Source: CAD feature listing. Evaluate the final solid. Frame: model axes, mm. A direction names the side the tool comes from. Give positions to 0.01 mm unless a question says otherwise; leave off trailing zeros. Loops run counter-clockwise (first coordinate to the right, second up) from the corner with the lowest first, then second, coordinate; pieces in that order, holes last. Notation, with made-up numbers: (4, 51) -> (22, 51) arc R10 cw to (22, 60) -> close; hole circle Ø7 at (55.25, 35). An arc over 180 degrees is marked (long way). Put each result on its own line as item: value.
```python
from build123d import *

# Parameters (mm, degrees)
SKETCH2_R             = 1.6
BOSS_EXTRUDE1_DEPTH   = 2
BOSS_EXTRUDE1_2_DEPTH = 2
BOSS_EXTRUDE2_DEPTH   = 12.7
SKETCH4_R             = 1.8
BOSS_EXTRUDE3_DEPTH   = 2
CHAMFER1_SIZE         = 2.54


with BuildPart() as part:
    # Sketch2 → Boss-Extrude1 (new body)
    with BuildSketch(Plane(origin=(0, 84.355025863, 0), x_dir=(1, 0, 0), z_dir=(0, 1, 0))):
        with BuildLine():
            Line((86.165130669, -169.940155685), (88.815130669, -169.940155685))
            ThreePointArc((88.815130669, -169.940155685), (90.611181893, -169.196206909), (91.355130669, -167.400155685))
            Line((91.355130669, -167.400155685), (91.355130669, -166.020155685))
            Line((91.355130669, -166.020155685), (94.293130669, -166.020155685))
            Line((94.293130669, -166.020155685), (94.293130669, -163.082155685))
            Line((94.293130669, -163.082155685), (94.293130669, -156.732155685))
            Line((94.293130669, -156.732155685), (86.165130669, -156.732155685))
            ThreePointArc((86.165130669, -156.732155685), (84.369079444, -157.47610446), (83.625130669, -159.272155685))
            Line((83.625130669, -159.272155685), (83.625130669, -167.400155685))
            ThreePointArc((83.625130669, -167.400155685), (84.369079444, -169.196206909), (86.165130669, -169.940155685))
        make_face()
        with Locations(Location((86.773356517, -166.898975693, 0), (0, 0, 270))):
            Circle(SKETCH2_R, mode=Mode.SUBTRACT)
        with Locations(Location((89.895511725, -160.090079663, 0), (0, 0, 270))):
            Circle(SKETCH2_R, mode=Mode.SUBTRACT)
    extrude(amount=BOSS_EXTRUDE1_DEPTH)



with BuildPart() as body_2:
    # Sketch2 → Boss-Extrude1 2 (new body)
    with BuildSketch(Plane(origin=(0, 84.355025863, 0), x_dir=(1, 0, 0), z_dir=(0, 1, 0))):
        with BuildLine():
            Line((113.995130669, -169.940155685), (116.645130669, -169.940155685))
            ThreePointArc((116.645130669, -169.940155685), (118.441181893, -169.196206909), (119.185130669, -167.400155685))
            Line((119.185130669, -167.400155685), (119.185130669, -159.272155685))
            ThreePointArc((119.185130669, -159.272155685), (118.441181893, -157.47610446), (116.645130669, -156.732155685))
            Line((116.645130669, -156.732155685), (108.517130669, -156.732155685))
            Line((108.517130669, -156.732155685), (108.517130669, -163.082155685))
            Line((108.517130669, -163.082155685), (108.517130669, -166.020155685))
            Line((108.517130669, -166.020155685), (111.455130669, -166.020155685))
            Line((111.455130669, -166.020155685), (111.455130669, -167.400155685))
            ThreePointArc((111.455130669, -167.400155685), (112.199079444, -169.196206909), (113.995130669, -169.940155685))
        make_face()
        with Locations(Location((116.03690482, -166.898975693, 0), (0, 0, 270))):
            Circle(SKETCH2_R, mode=Mode.SUBTRACT)
        with Locations(Location((112.914749612, -160.090079663, 0), (0, 0, 270))):
            Circle(SKETCH2_R, mode=Mode.SUBTRACT)
    extrude(amount=BOSS_EXTRUDE1_2_DEPTH)


with BuildPart() as part_1:
    add(part.part)

    add(body_2.part)  # Boss-Extrude2 merges body 2
    # Sketch3 → Boss-Extrude2 (add)
    with BuildSketch(Plane(origin=(0, 86.355025863, 0), x_dir=(1, 0, 0), z_dir=(0, 1, 0))):
        with BuildLine():
            Line((108.517130669, -158.002155685), (108.517130669, -156.732155685))
            Line((108.517130669, -156.732155685), (94.293130669, -156.732155685))
            Line((94.293130669, -156.732155685), (86.165130669, -156.732155685))
            ThreePointArc((86.165130669, -156.732155685), (84.369079444, -157.47610446), (83.625130669, -159.272155685))
            Line((83.625130669, -159.272155685), (83.625130669, -164.352155685))
            Line((83.625130669, -164.352155685), (87.435130669, -164.352155685))
            Line((87.435130669, -164.352155685), (87.435130669, -158.002155685))
            Line((87.435130669, -158.002155685), (108.517130669, -158.002155685))
        make_face()
        with BuildLine():
            Line((115.375130669, -164.352155685), (119.185130669, -164.352155685))
            Line((119.185130669, -164.352155685), (119.185130669, -159.272155685))
            ThreePointArc((119.185130669, -159.272155685), (118.441181893, -157.47610446), (116.645130669, -156.732155685))
            Line((116.645130669, -156.732155685), (108.517130669, -156.732155685))
            Line((108.517130669, -156.732155685), (108.517130669, -158.002155685))
            Line((108.517130669, -158.002155685), (115.375130669, -158.002155685))
            Line((115.375130669, -158.002155685), (115.375130669, -164.352155685))
        make_face()
    extrude(amount=BOSS_EXTRUDE2_DEPTH)

    # Sketch4 → Boss-Extrude3 (add)
    with BuildSketch(Plane(origin=(0, 99.055025863, 0), x_dir=(1, 0, 0), z_dir=(0, 1, 0))):
        with BuildLine():
            Line((83.625130669, -164.352155685), (83.625130669, -191.022155685))
            Line((83.625130669, -191.022155685), (119.185130669, -191.022155685))
            Line((119.185130669, -191.022155685), (119.185130669, -164.352155685))
            Line((119.185130669, -164.352155685), (119.185130669, -159.272155685))
            ThreePointArc((119.185130669, -159.272155685), (118.441181893, -157.47610446), (116.645130669, -156.732155685))
            Line((116.645130669, -156.732155685), (86.165130669, -156.732155685))
            ThreePointArc((86.165130669, -156.732155685), (84.369079444, -157.47610446), (83.625130669, -159.272155685))
            Line((83.625130669, -159.272155685), (83.625130669, -164.352155685))
        make_face()
        with Locations(Location((93.405130669, -184.164155685, 0), (0, 0, 270))):
            Circle(SKETCH4_R, mode=Mode.SUBTRACT)
        with Locations(Location((109.405130669, -184.164155685, 0), (0, 0, 270))):
            Circle(SKETCH4_R, mode=Mode.SUBTRACT)
    extrude(amount=BOSS_EXTRUDE3_DEPTH)

    # Chamfer1
    chamfer1_edges = [part_1.edges().sort_by_distance(p)[0] for p in [
        (85.530130669, 99.055025863, 164.352155685),
        (87.435130669, 99.055025863, 161.177155685),
        (101.405130669, 99.055025863, 158.002155685),
        (115.375130669, 99.055025863, 161.177155685),
        (117.280130669, 99.055025863, 164.352155685),
    ]]
    chamfer(chamfer1_edges, length=CHAMFER1_SIZE)


solid = part_1.part
```
(1) Reachability of faces 1 (the cylindrical face through (114.6, 85.3, 167.6)), 2 (the flat face through (116.671, 97.803, 165.64)), 3 (the flat face through (88.72, 97.8, 162.51)), 4 (the cylindrical face through (90.591, 85.341, 169.216)), 5 (the flat face through (108.517, 85, 161)) from +Z, -Z, +X, -X, +Y, -Y: full face, straight path, thin tool, end or side. Return the list, or none.
Calculated:
face 1: -Y
face 2: +Z, +X, -X
face 3: +Z
face 4: +Z, -Y
face 5: +Z, -Z, -Y
(2) Line query: probe 1 along X at (y, z) = (99.25, 183); probe 2 along X at (y, z) = (89, 162.5); probe 3 along X at (y, z) = (85.5, 161.5). Output: solid intervals per line, ascending. Write a range as from..to.
Calculated:
probe 1: x = 83.63..92.03, 94.78..108.03, 110.78..119.19
probe 2: x = 83.63..87.44, 115.38..119.19
probe 3: x = 83.63..89.14, 90.65..94.29, 108.52..112.16, 113.67..119.19
(3) First-contact query: P1, Ø0.6, axis at x = 115.5, y = 85, coming from the +Z side; P2, Ø4, axis at x = 117, y = 91, coming from the +Z side; P3, Ø1, axis at x = 92, y = 90.5, coming from the +Z side; P4, Ø4, axis at x = 116.04, z = 166.9, coming from the -Y side (3 decimals). Flat tips, straight axial feed; report the tip coordinate or a pass-through.
Calculated:
P1: stops at z = 169.94
P2: stops at z = 164.35
P3: stops at z = 158
P4: stops at y = 84.355
(4) Section C-C on z = 169. Return loops of the section in (x, y).
Calculated:
outline: (83.63, 99.06) -> (119.19, 99.06) -> (119.19, 101.06) -> (83.63, 101.06) -> close; (84.19, 84.36) -> (90.79, 84.36) -> (90.79, 86.36) -> (84.19, 86.36) -> close; (112.02, 84.36) -> (118.62, 84.36) -> (118.62, 86.36) -> (112.02, 86.36) -> close
(5) Section A-A on y = 94.75. Return loops of the section in (x, z).
Calculated:
outline: (83.63, 159.27) arc R2.54 ccw to (86.17, 156.73) -> (116.65, 156.73) arc R2.54 ccw to (119.19, 159.27) -> (119.19, 164.35) -> (115.38, 164.35) -> (115.38, 158) -> (87.44, 158) -> (87.44, 164.35) -> (83.63, 164.35) -> close
(6) Section B-B on x = 103. Return loops of the section in (y, z).
Calculated:
outline: (86.36, 156.73) -> (101.06, 156.73) -> (101.06, 191.02) -> (99.06, 191.02) -> (99.06, 160.54) -> (96.52, 158) -> (86.36, 158) -> close
(7) Draft query along Z for faces 6 (the flat face through (101, 100, 191.022)), 7 (the flat face through (90, 86.355, 164)), 8 (the cylindrical face through (113.996, 85.341, 158.911)). Return one class per face: released by +Z, released by -Z, zero draft, split by the parting line, or undercut.
Calculated:
face 6: released by +Z
face 7: zero draft
face 8: undercut
(8) Section D-D on x = 92.5. Return loops of the section in (y, z), then the cut area to 3 significant figures.
Calculated:
outline: (84.36, 156.73) -> (101.06, 156.73) -> (101.06, 182.61) -> (99.06, 182.61) -> (99.06, 160.54) -> (96.52, 158) -> (86.36, 158) -> (86.36, 166.02) -> (84.36, 166.02) -> close; (99.06, 185.72) -> (101.06, 185.72) -> (101.06, 191.02) -> (99.06, 191.02) -> close
area: 100 mm²
